Source: CAD feature listing. Evaluate the final solid. Frame: model axes, mm. A direction names the side the tool comes from. Coordinates: 2 decimals unless noted, no trailing zeros. Order: outer loops, then holes, each group sorted by start corner. A loop starts at its lowest first (then second) coordinate and runs counter-clockwise, first axis right, second up. Notation, with made-up numbers: (-30.5, 51) -> (27.5, 51) arc R33 cw to (27.5, 89) -> close; hole circle Ø3 at (63.5, -34.5). An arc over 180 degrees is marked (long way). Write item = value, one per line. Start each with the question number.
Item 1: Section query C-C (z = 606.5). Output: boundary loops of the cut face in (x, y).
Item 2: Section query B-B (z = 183). Output: boundary loops of the cut face in (x, y), then the cut area to 3 significant figures.
Item 3: Set-up query: faces 1 (the flat face through (3, -45, 475)), 2 (the flat face through (-3, 199, 871)), 3 (the flat face through (-207, -190, 210)). Return all of +Z, -Z, +X, -X, +Y, -Y with unobstructed straight access to the full face (end or side cutting, diameter ignored); none if empty.
Item 4: Ray query, line 1 along Z through (x, y) = (206, -46); line 2 along Y through (x, z) = (-1, 904.5); line 3 along Y through (x, z) = (-94.5, 770.5). Return the intervals inside material, ascending. Write a range as [from, to].
Item 5: Contact query for flat-ended pins moving along their axis: pin 1 (8 mm diameter, centred on x = 43.5, y = -70, fed in from +Z); pin 2 (1 mm diameter, centred on x = -154, y = 172, fed in from -Z); pin 3 (17.5 mm diameter, centred on x = -213, z = 155, fed in from +Y); pin 4 (12 mm diameter, centred on y = 154.5, z = 636.5, fed in from -X). Output: stop coordinate, or through.
Item 6: Mould query, pull axis Y, two halves, no side actions, for faces 4 (the flat face through (3, -28, 425)), 5 (the flat face through (1, 175, 432)), 6 (the flat face through (-2.66, 185.854, 746.693)). Classes: released by +Y, released by -Y, zero draft, split by the parting line, or undercut.
Item 7: Section query D-D (y = -91). Output: boundary loops of the cut face in (x, z), then the cut area to 3 significant figures.
Item 8: Section query A-A (x = 54.5). Output: boundary loops of the cut face in (y, z).
```python
from build123d import *

# Parameters (mm, degrees)
F0_W     = 450
F0_H     = 450
F1_DEPTH = 950
F2_W     = 330
F2_H     = 425
F2_W_2   = 50
F3_DEPTH = 450.001
F4_W     = 380
F4_H     = 425
F5_DEPTH = 450.001
F6_W     = 380
F6_H     = 75
F6_H_2   = 275
F7_DEPTH = 134.2592361444


with BuildPart() as f1:
    # F0 (on Top) → F1 (new body)
    with BuildSketch(Plane.XY):
        Rectangle(F0_W, F0_H)
    extrude(amount=F1_DEPTH)

    # F2 (on face) → F3 (cut, through all)
    with BuildSketch(Plane.YZ.offset(225)):
        Polygon((225, 473.0396032333), (225, 475), (175, 475), (175, 425), (225, 425), align=None)
        Polygon((-225, 475), (140, 475), (190, 950), (-225, 950), (-225, 495.331287384), (-225, 493.3708906174), align=None)
        with Locations((-25, 212.5)):
            Rectangle(F2_W, F2_H)
        with Locations((200, 212.5)):
            Rectangle(F2_W_2, F2_H)
        Polygon((175, 475), (225, 475), (225, 950), align=None)
    extrude(amount=-F3_DEPTH, mode=Mode.SUBTRACT)

    # F4 (on face) → F5 (cut, through all)
    with BuildSketch(Plane.XZ.offset(225)):
        with Locations((0, 212.5)):
            Rectangle(F4_W, F4_H)
    extrude(amount=-F5_DEPTH, mode=Mode.SUBTRACT)

    # F6 (on face) → F7 (cut, through all)
    with BuildSketch(Plane(origin=(0, 89.0136986301, -9.3698630137), x_dir=(1, 0, 0), z_dir=(0, -0.9945054529, 0.1046847845))):
        with Locations((0, 849.5459599702)):
            Rectangle(F6_W, F6_H)
        with Locations((0, 624.5459599702)):
            Rectangle(F6_W, F6_H_2)
    extrude(amount=-F7_DEPTH, mode=Mode.SUBTRACT)


solid = f1.part
```
Computed:
q1.outline = (-225, 153.84) -> (-190, 153.84) -> (-190, 188.84) -> (-225, 188.84) -> close; (190, 153.84) -> (225, 153.84) -> (225, 188.84) -> (190, 188.84) -> close
q2.outline = (-225, -225) -> (-190, -225) -> (-190, -190) -> (-225, -190) -> close; (-225, 140) -> (-190, 140) -> (-190, 175) -> (-225, 175) -> close; (190, -225) -> (225, -225) -> (225, -190) -> (190, -190) -> close; (190, 140) -> (225, 140) -> (225, 175) -> (190, 175) -> close
q2.area = 4,900 mm^2
q3.face_1 = +Z, +X, -X, -Y
q3.face_2 = -Y
q3.face_3 = -Z, +X, -X
q4.line_1 = [425, 475]
q4.line_2 = [185.21, 220.21]
q4.line_3 = [171.11, 206.11]
q5.pin_1 = 475
q5.pin_2 = 425
q5.pin_3 = 175
q5.pin_4 = -225
q6.face_4 = undercut
q6.face_5 = released by +Y
q6.face_6 = released by -Y
q7.outline = (-225, 425) -> (225, 425) -> (225, 475) -> (-225, 475) -> close
q7.area = 22,500 mm^2
q8.outline = (-225, 425) -> (175, 425) -> (175, 471.32) -> (140, 475) -> (-225, 475) -> close; (168.79, 748.49) -> (203.4, 744.85) -> (208.64, 794.57) -> (174.02, 798.21) -> close; (181.87, 872.8) -> (216.49, 869.16) -> (225, 950) -> (190, 950) -> close
